Job drawing, mm, ordinate dimensions from the low corner. One solid piece. A direction names the side the tool comes from. Coordinates: 2 decimals unless noted, no trailing zeros. Write each loop counter-clockwise with the first axis right and the second up, starting at its lowest first coordinate (ties: lowest second). Pieces come first, ordered by that corner, then holes. Notation, with made-up numbers: (-18, -39.75) - (-5, -39.75) arc R28 cw to (-5, -8.75) - close; hole circle Ø4 at (-9.75, 53). An arc over 180 degrees is marked (long way). Put each result on its own line as item: value. Start each with the question number.
1. Which spindle directions (+Z, -Z, +X, -X, +Y, -Y) get a long thin tool onto all of the face, cutting with end or side? Do the marked faces 1 and 2. Say none if no direction does.
2. Saw through at A-A, the plane y = 1. Write the cut outline in (x, z).
3. Saw through at C-C, the plane z = 38.1. Write the cut outline in (x, y).
4. Saw through at D-D, the plane y = 15. Write the cut outline in (x, z) (1 decimal).
5. Saw through at B-B, the plane y = 6.5. Give the number of separate pieces and of enclosed holes in the cut face.
6. Drop flat-ended pins along their axis: P1, Ø1, axis at x = 65, y = 14.5, coming from the +Z side (1 decimal); P2, Ø9, axis at x = 71.12, z = 5.08, coming from the +Y side; P3, Ø3, axis at x = 34, y = 14.5, coming from the +Z side. Give the stop position or say it passes through.
7. Drill centre lines: L1, parallel to X at y = 7.5, z = 55.5 (1 decimal); L2, parallel to Z at x = 71.12, y = 3.75. Where is each one in solid material? Low to high. Write a range as from..to.
8. Pull direction Z, two halves, no side cores. Call the marked faces 3, 4 and 5: released by +Z, released by -Z, zero draft, split by the parting line, or undercut.
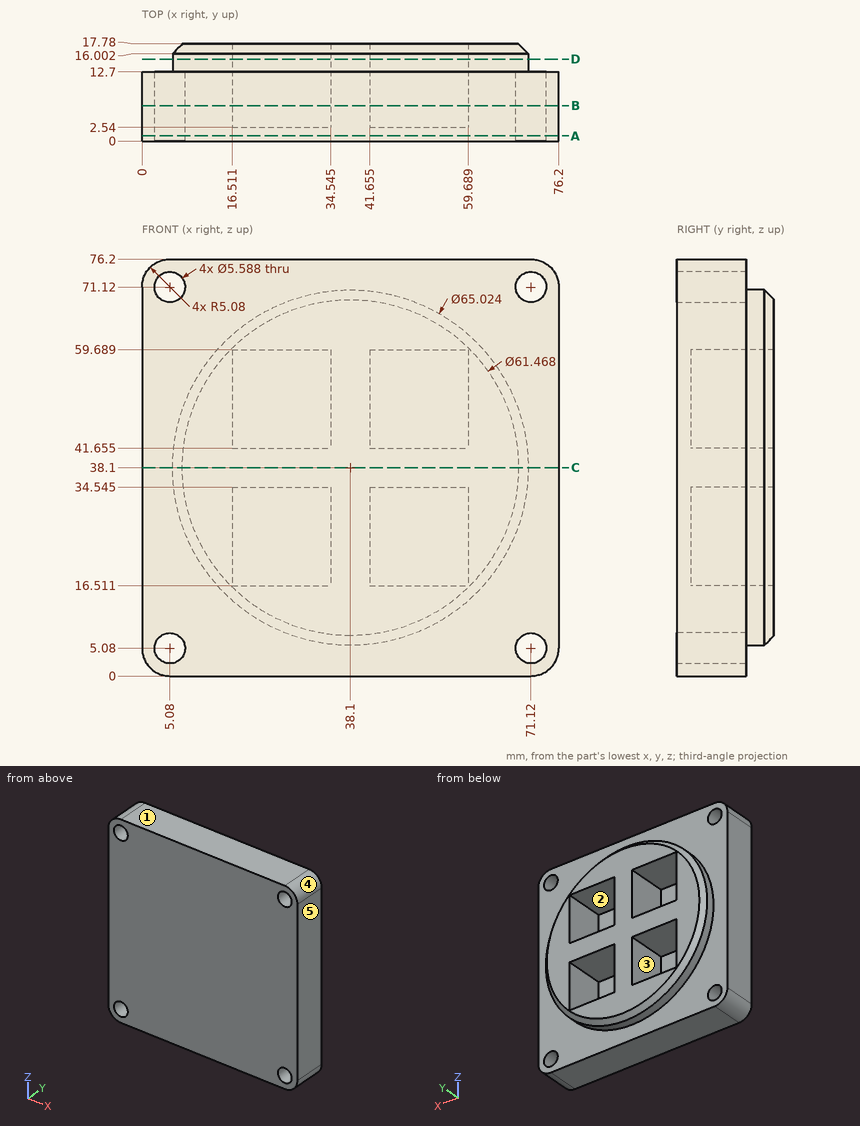
Final values:
1. face 1: +Z, +X, -X, +Y, -Y
1. face 2: +Y
2. outline: (0, 5.08) arc R5.08 ccw to (5.08, 0) - (71.12, 0) arc R5.08 ccw to (76.2, 5.08) - (76.2, 71.12) arc R5.08 ccw to (71.12, 76.2) - (5.08, 76.2) arc R5.08 ccw to (0, 71.12) - close; hole circle Ø5.59 at (5.08, 5.08); hole circle Ø5.59 at (5.08, 71.12); hole circle Ø5.59 at (71.12, 5.08); hole circle Ø5.59 at (71.12, 71.12)
3. outline: (0, 0) - (76.2, 0) - (76.2, 12.7) - (70.61, 12.7) - (70.61, 16) - (68.83, 17.78) - (7.37, 17.78) - (5.59, 16) - (5.59, 12.7) - (0, 12.7) - close
4. outline: circle Ø65 at (38.1, 38.1); hole (16.5, 16.5) - (34.5, 16.5) - (34.5, 34.5) - (16.5, 34.5) - close; hole (16.5, 41.7) - (34.5, 41.7) - (34.5, 59.7) - (16.5, 59.7) - close; hole (41.7, 16.5) - (59.7, 16.5) - (59.7, 34.5) - (41.7, 34.5) - close; hole (41.7, 41.7) - (59.7, 41.7) - (59.7, 59.7) - (41.7, 59.7) - close
5. separate pieces: 1
5. enclosed holes: 8
6. P1: stops at z = 57.1
6. P2: stops at y = 12.7
6. P3: stops at z = 70.51
7. L1: x = 0..16.5, 34.5..41.7, 59.7..76.2
7. L2: z = 0..2.29, 7.87..68.33, 73.91..76.2
8. face 3: undercut
8. face 4: released by +Z
8. face 5: zero draft
